Autodesk Fusion 360 part; units mm, degrees
sketch "Sketch1" plane through (0, 0, 0) normal (0, 0, 1) x (1, 0, 0)
  line L0 (-63.395, 42.575) -> (63.395, 42.575)
  line L1 (63.395, 42.575) -> (63.395, -42.575)
  line L2 (63.395, -42.575) -> (-63.395, -42.575)
  line L3 (-63.395, -42.575) -> (-63.395, 42.575)
  line L4 (-63.395, 42.575) -> (63.395, -42.575) construction
  line L5 (63.395, 42.575) -> (-63.395, -42.575) construction
  dimension "d1" = 126.79
  dimension "d2" = 85.15
sketch "Sketch2" plane through (0, 0, 0) normal (0, 1, 0) x (1, 0, 0)
sketch "Sketch3" plane through (0, 0, 0) normal (0, 0, 1) x (1, 0, 0)
  line L0 (66.395, -45.575) -> (-66.395, -45.575)
  line L1 (-66.395, -45.575) -> (-66.395, 45.575)
  line L2 (-66.395, 45.575) -> (66.395, 45.575)
  line L3 (66.395, 45.575) -> (66.395, -45.575)
  line L4 (66.395, -45.575) -> (-66.395, 45.575) construction
  line L5 (-66.395, -45.575) -> (66.395, 45.575) construction
  dimension "d3" = 132.79
  dimension "d4" = 91.15
extrude "Extrude1" add sketch "Sketch3" along normal blind 28
shell "Shell1" thickness 3 removed faces 1 at (-22.1317, 15.1917, 28)
extrude "Extrude2" add sketch "Sketch1" against normal blind 4
extrude "Extrude3" add 1 faces at (-21.1317, 14.1917, -4) along direction (0, 0, -1) blind 3.9
For this review, take the finished solid that the model builds, in its own axes (mm). A direction names the side the tool comes from. Coordinates: 2 decimals unless noted, no trailing zeros. Loops run counter-clockwise (first coordinate to the right, second up) from the corner with the lowest first, then second, coordinate; pieces in that order, holes last. Notation, with made-up numbers: (29.5, 31.5) - (74.5, 31.5) arc R14 ccw to (74.5, 44.5) - close; hole circle Ø10 at (83.25, 1). An arc over 180 degrees is marked (long way). Use a Markdown table: item, result. Add a question column.
Item 1: We need section C-C (x = 40.5). Give the boundary of the cut face in (y, z) (3 decimals).
Item 2: We need section B-B (y = -35). Give the boundary of the cut face in (x, z) (3 decimals), and give its area (3 significant figures).
Item 3: For line 1 (X direction, y = -6, z = 14) (3 decimals); line 2 (Y direction, x = 39.5, z = 10.5) (3 decimals); line 3 (X direction, y = -5, z = -3) (3 decimals), list the stretches that pass through material, from the lowest coordinate up.
Item 4: Insertion check: pin 1 Ø8.5 at (y, z) = (16.5, -4) entering from +X (3 decimals); pin 2 Ø4 at (x, z) = (10, -4) entering from -Y (3 decimals); pin 3 Ø1 at (x, y) = (-49, -36) entering from +Z; pin 4 Ø6.5 at (x, z) = (4, -4.5) entering from +Y (3 decimals). Each pin has a flat end and moves straight along its axis. Give the tip position at first contact, or say it passes through.
Item 5: We need section A-A (z = 14.5). Give the boundary of the cut face in (x, y) (3 decimals), and give its area (3 significant figures).
Item 6: Tool access review of faces 1 (the face through (-63.395, -1, -4)), 2 (the face through (-1, 42.575, -4)), 3 (the face through (63.395, 1, -4)), 4 (the face through (1, -42.575, -4)), 5 (the face through (-1, 42.575, 15)): name each direction out of +Z, -Z, +X, -X, +Y, -Y from which nothing blocks a thin tool from reaching the whole face with its end or side.
Results list:
| question | item | result |
|---|---|---|
| 1 | outline | (-45.575, 0) - (-42.575, 0) - (-42.575, -7.9) - (42.575, -7.9) - (42.575, 0) - (45.575, 0) - (45.575, 28) - (42.575, 28) - (42.575, 3) - (-42.575, 3) - (-42.575, 28) - (-45.575, 28) - close |
| 2 | outline | (-66.395, 0) - (-63.395, 0) - (-63.395, -7.9) - (63.395, -7.9) - (63.395, 0) - (66.395, 0) - (66.395, 28) - (63.395, 28) - (63.395, 3) - (-63.395, 3) - (-63.395, 28) - (-66.395, 28) - close |
| 2 | area | 1,550 mm^2 |
| 3 | line 1 | x = -66.395 to -63.395, 63.395 to 66.395 |
| 3 | line 2 | y = -45.575 to -42.575, 42.575 to 45.575 |
| 3 | line 3 | x = -63.395 to 63.395 |
| 4 | pin 1 | stops at x = 66.395 |
| 4 | pin 2 | stops at y = -42.575 |
| 4 | pin 3 | stops at z = 3 |
| 4 | pin 4 | stops at y = 42.575 |
| 5 | outline | (-66.395, -45.575) - (66.395, -45.575) - (66.395, 45.575) - (-66.395, 45.575) - close; hole (-63.395, -42.575) - (63.395, -42.575) - (63.395, 42.575) - (-63.395, 42.575) - close |
| 5 | area | 1,310 mm^2 |
| 6 | face 1 | -Z, -X, +Y, -Y |
| 6 | face 2 | -Z, +X, -X, +Y |
| 6 | face 3 | -Z, +X, +Y, -Y |
| 6 | face 4 | -Z, +X, -X, -Y |
| 6 | face 5 | +Z |
